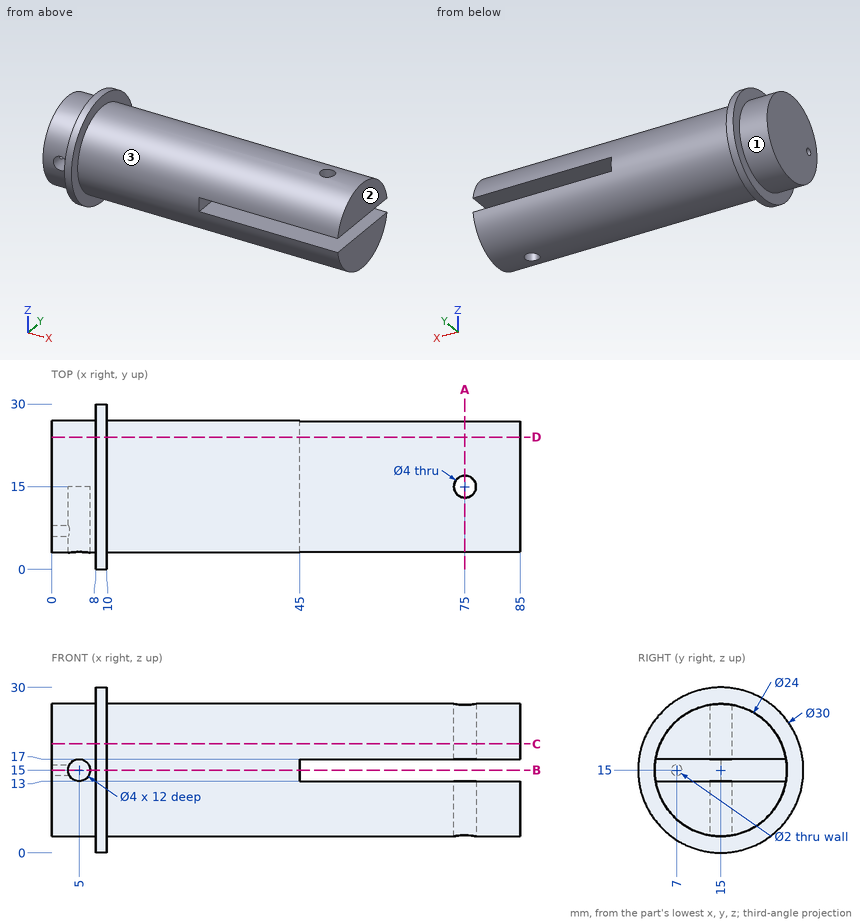
Input: dimensioned drawing with shaded views. Units: mm. Origin: part minimum x, y, z. A direction names the side the tool comes from. Coordinates: 2 decimals unless noted, no trailing zeros. Order: outer loops, then holes, each group sorted by start corner. A loop starts at its lowest first (then second) coordinate and runs counter-clockwise, first axis right, second up. Notation, with made-up numbers: (64, 37.25) - (117, 37.25) arc R13 cw to (117, 62.25) - close; hole circle Ø4 at (53, 87). An arc over 180 degrees is marked (long way). Put each result on its own line as item: value.
1. Cut plane C-C on z = 19.75. Return the cut outline in (x, y), then the cut area to 3 significant figures.
Report:
outline: (0, 3.98) - (8, 3.98) - (8, 0.77) - (10, 0.77) - (10, 3.98) - (85, 3.98) - (85, 26.02) - (10, 26.02) - (10, 29.23) - (8, 29.23) - (8, 26.02) - (0, 26.02) - close; hole circle Ø4 at (75, 15)
area: 1,870 mm2
2. Reachability of the marked faces 1, 2 and 3 from +Z, -Z, +X, -X, +Y, -Y: full face, straight path, thin tool, end or side. Return the list, or none.
Report:
face 1: -X
face 2: +Z, -Z, +X, +Y, -Y
face 3: +X
3. Line query: line 1 along X through (y, z) = (15, 5.75); line 2 along Z through (x, y) = (0.75, 7); line 3 along Y through (x, z) = (75, 10.25). Output: solid intervals per line, ascending.
Report:
line 1: x = 0 to 73, 77 to 85
line 2: z = 6.06 to 14, 16 to 23.94
line 3: y = 3.98 to 13, 17 to 26.02
4. Cut plane A-A on x = 75. Return the cut outline in (y, z).
Report:
outline: (3.17, 13) arc R12 ccw to (13, 3.17) - (13, 13) - close; (3.17, 17) - (13, 17) - (13, 26.83) arc R12 ccw to start; (17, 3.17) arc R12 ccw to (26.83, 13) - (17, 13) - close; (17, 17) - (26.83, 17) arc R12 ccw to (17, 26.83) - close
5. Cut plane B-B on z = 15. Return the cut outline in (x, y).
Report:
outline: (0, 3) - (3, 3) - (3, 6) - (0, 6) - close; (0, 8) - (3, 8) - (3, 15) - (7, 15) - (7, 3) - (8, 3) - (8, 0) - (10, 0) - (10, 3) - (45, 3) - (45, 27) - (10, 27) - (10, 30) - (8, 30) - (8, 27) - (0, 27) - close
6. Cut plane D-D on y = 24. Return the cut outline in (x, z), then the cut area to 3 significant figures.
Report:
outline: (0, 7.06) - (8, 7.06) - (8, 3) - (10, 3) - (10, 7.06) - (85, 7.06) - (85, 13) - (45, 13) - (45, 17) - (85, 17) - (85, 22.94) - (10, 22.94) - (10, 27) - (8, 27) - (8, 22.94) - (0, 22.94) - close
area: 1,210 mm2
7. Contact query for flat-ended pins moving along their axis: pin 1 Ø4 at (x, y) = (23, 8.5) entering from +Z; pin 2 Ø1 at (x, y) = (48.5, 20.5) entering from +Z; pin 3 Ø2.5 at (x, z) = (5, 15) entering from +Y; pin 4 Ø2.5 at (x, y) = (75, 15) entering from -Z. Output: stop coordinate, or through.
Report:
pin 1: stops at z = 26.12
pin 2: stops at z = 25.91
pin 3: stops at y = 27
pin 4: passes through
